The listing builds one solid part. Answer for the finished solid, in the listing's coordinates (mm). Coordinates: 2 decimals unless noted, no trailing zeros. Write each question's results on one line, items separated by ' | '. Start each with the question number.
(1) Straight lines are drawn through the part: L1, parallel to X at y = -35.5, z = 10; L2, parallel to Z at x = 11, y = -65; L3, parallel to X at y = -123.5, z = -11. For each, find the intervals that lie inside material, in ascending order.
(2) Given pin 1 (4 mm diameter, centred on x = 13.5, y = -122.5, fed in from -Z); pin 2 (6 mm diameter, centred on x = -12.5, y = -72.5, fed in from -Z); pin 3 (4 mm diameter, centred on x = -7.5, z = 0, fed in from +Y); pin 4 (10 mm diameter, centred on x = -12, y = -93.5, fed in from -Z), each flat-ended and moving along its own axis, determine where each tip first touches the part or whether it passes through.
(3) Determine the mould class of faces 1 (the face through (0, -69, 20)), 2 (the face through (-20, -85, 5)), 3 (the face through (0, -138, 19.5)) for opening direction X: +X half, -X half, draft (parallel to the pull), parting line (faces both ways), or undercut.
(4) The part is cut by section A-A, the plane z = -2.5. Count the separate pieces of the cut face and the enclosed holes in it, then the cut area to 3 significant figures.
```python
from build123d import *

# Parameters (mm, degrees)
F0_W      = 34
F0_H      = 1.332180649
F0_W_2    = 3
F0_H_2    = 30
F1_DEPTH  = 140
F3_DEPTH  = 50
F4_DEPTH  = 40
F5_T      = -0.5
F7_REACH  = 112.8020988928
F9_DEPTH  = 40
F11_DEPTH = 1000
F12_R     = 6.3171610822
F13_DEPTH = 140


# Not quite as in the source:
# - a feature names something its author has since deleted; it is built from what else it names


with BuildPart() as f1:
    # F0 (on Front) → F1 (new body)
    with BuildSketch(Plane.XZ):
        Polygon((20, 20), (17, 20), (17, 18.832180649), (17, 17.5), (17, 15), (20, 15), align=None)
        Polygon((15, 20), (-15, 20), (-17, 20), (-17, 18.832180649), (17, 18.832180649), (17, 20), align=None)
        with Locations((0, 18.1660903245)):
            Rectangle(F0_W, F0_H)
        Polygon((17, 17.5), (-17, 17.5), (-17, 15), (-17, -15), (-15, -15), (15, -15), (17, -15), (17, 15), align=None)
        Polygon((-18.5, 15), (-20, 15), (-20, -11.8550653383), (-20, -15), (-18.5, -15), (-18.5, -5.2632528394), (-18.5, -3.2632528394), (-18.5, 2.7367471606), (-18.5, 4.7367471606), align=None)
        with Locations((18.5, 0)):
            Rectangle(F0_W_2, F0_H_2)
        with BuildLine():
            Line((-15, -20), (15, -20))
            Line((15, -20), (15, -17.5))
            Line((15, -17.5), (11.391207267, -17.5))
            ThreePointArc((11.391207267, -17.5), (10.2485464886, -18.6426607784), (9.1058857102, -17.5))
            Line((9.1058857102, -17.5), (7.9234171988, -17.5))
            ThreePointArc((7.9234171988, -17.5), (5.948765669, -19.4746515298), (3.9741141393, -17.5))
            Line((3.9741141393, -17.5), (2.0740236579, -17.5))
            ThreePointArc((2.0740236579, -17.5), (0, -19.5740236579), (-2.0740236579, -17.5))
            Line((-2.0740236579, -17.5), (-3.9741141393, -17.5))
            ThreePointArc((-3.9741141393, -17.5), (-5.948765669, -19.4746515298), (-7.9234171988, -17.5))
            Line((-7.9234171988, -17.5), (-9.1058857102, -17.5))
            ThreePointArc((-9.1058857102, -17.5), (-10.2485464886, -18.6426607784), (-11.391207267, -17.5))
            Line((-11.391207267, -17.5), (-15, -17.5))
            Line((-15, -17.5), (-15, -20))
        make_face()
        Polygon((20, -20), (20, -15), (17, -15), (15, -15), (15, -17.5), (15, -20), align=None)
        Polygon((-17, -15), (-17, 15), (-18.5, 15), (-18.5, 4.7367471606), (-18.5, 2.7367471606), (-18.5, -3.2632528394), (-18.5, -5.2632528394), (-18.5, -15), align=None)
        Polygon((-15, -17.5), (-15, -15), (-16.767766953, -16.767766953), (-17.5, -17.5), (-15, -20), align=None)
        Polygon((-15, -15), (-17, -15), (-18.5, -15), (-20, -15), (-17.5, -17.5), (-16.767766953, -16.767766953), align=None)
        Polygon((-17, 18.832180649), (-17, 20), (-20, 20), (-20, 15), (-18.5, 15), (-17, 15), (-17, 17.5), align=None)
        Polygon((-17.5, -17.5), (-20, -15), (-20, -20), (-15, -20), align=None)
        with BuildLine():
            Line((3.9741141393, -17.5), (7.9234171988, -17.5))
            ThreePointArc((7.9234171988, -17.5), (5.948765669, -15.5253484702), (3.9741141393, -17.5))
        make_face()
        with BuildLine():
            ThreePointArc((3.9741141393, -17.5), (5.948765669, -19.4746515298), (7.9234171988, -17.5))
            Line((7.9234171988, -17.5), (3.9741141393, -17.5))
        make_face()
        with BuildLine():
            ThreePointArc((9.1058857102, -17.5), (10.2485464886, -18.6426607784), (11.391207267, -17.5))
            Line((11.391207267, -17.5), (9.1058857102, -17.5))
        make_face()
        with BuildLine():
            Line((9.1058857102, -17.5), (11.391207267, -17.5))
            ThreePointArc((11.391207267, -17.5), (10.2485464886, -16.3573392216), (9.1058857102, -17.5))
        make_face()
        with BuildLine():
            ThreePointArc((2.0740236579, -17.5), (0, -15.4259763421), (-2.0740236579, -17.5))
            Line((-2.0740236579, -17.5), (2.0740236579, -17.5))
        make_face()
        with BuildLine():
            Line((2.0740236579, -17.5), (-2.0740236579, -17.5))
            ThreePointArc((-2.0740236579, -17.5), (0, -19.5740236579), (2.0740236579, -17.5))
        make_face()
        with BuildLine():
            Line((-3.9741141393, -17.5), (-7.9234171988, -17.5))
            ThreePointArc((-7.9234171988, -17.5), (-5.948765669, -19.4746515298), (-3.9741141393, -17.5))
        make_face()
    extrude(amount=F1_DEPTH)


with BuildPart() as f1b:
    # F0 (on Front) → F1, piece 2 (new body)
    with BuildSketch(Plane.XZ):
        with BuildLine():
            ThreePointArc((-9.1058857102, -17.5), (-10.2485464886, -16.3573392216), (-11.391207267, -17.5))
            Line((-11.391207267, -17.5), (-9.1058857102, -17.5))
        make_face()
    extrude(amount=F1_DEPTH)


with BuildPart() as f3_tool:
    # F2 (on face) → F3 (new body)
    with BuildSketch(Plane.YZ.offset(20)):
        Polygon((0, 0), (-132.0431083441, -20), (0, -20), align=None)
    extrude(amount=-F3_DEPTH)


with BuildPart() as f1_1:
    add(f1.part)

    # F3: cut by f3_tool
    add(f3_tool.part, mode=Mode.SUBTRACT)



with BuildPart() as f1b_1:
    add(f1b.part)

    # F3: cut by f3_tool
    add(f3_tool.part, mode=Mode.SUBTRACT)


with BuildPart() as f1_2:
    add(f1_1.part)

    add(f1b_1.part)  # F4 merges F1b
    # F2 (on face) → F4 (join)
    with BuildSketch(Plane.YZ.offset(20)):
        Polygon((-133.1249161121, -12.857736984), (-132.0431083441, -20), (0, 0), (0, 7.3061197718), align=None)
        Polygon((-140, -20), (-132.0431083441, -20), (-133.1249161121, -12.857736984), (-140, -13.8990762821), align=None)
    extrude(amount=-F4_DEPTH)

    # F5
    f5_openings = [f1_2.faces().sort_by_distance(p)[0] for p in [
        (0, -140, 0),
    ]]
    offset(amount=F5_T, openings=f5_openings)

    f7_end = Plane(origin=(0, -66.021554172, -10), x_dir=(0, -0.988722747, -0.1497575692), z_dir=(0, 0.1497575692, -0.988722747))
    # F6 (on face) → F7 (join, up to a plane its end follows)
    with BuildSketch(Plane.XY.offset(20)):
        Polygon((0, -70), (-0.1507168075, -70), (0, -70.5315142328), (0.1507168075, -70), align=None)
        Polygon((0, -69.4684857672), (-0.1507168075, -70), (0, -70), (0.1507168075, -70), align=None)
        Polygon((0.1507168075, -70), (0, -70.5315142328), (19.6985663849, -140), (20, -140), align=None)
        Polygon((0, -70.5315142328), (-0.1507168075, -70), (-20, -140), (-19.6985663849, -140), align=None)
        Polygon((19.6985663849, 0), (0, -69.4684857672), (0.1507168075, -70), (20, 0), align=None)
        Polygon((-19.6985663849, 0), (-20, 0), (-0.1507168075, -70), (0, -69.4684857672), align=None)
    f7_long = extrude(amount=-F7_REACH, mode=Mode.PRIVATE)
    add(split(f7_long, bisect_by=f7_end, keep=Keep.BOTTOM, mode=Mode.PRIVATE))

    # F8 (on face) → F9 (join, through all)
    with BuildSketch(Plane.YZ.offset(20)):
        Polygon((-47.3704106226, 6.7672015175), (-46.6666666667, 6.6666666667), (-45.9831301115, 6.8619628253), (-46.6868740675, 6.9624976761), align=None)
        Polygon((-46.6868740675, 6.9624976761), (-45.9831301115, 6.8619628253), (0, 20), (-1.0556159339, 20), align=None)
        Polygon((-140, 20), (-47.3704106226, 6.7672015175), (-46.6868740675, 6.9624976761), (-137.9493903346, 20), align=None)
        Polygon((-45.9831301115, 6.8619628253), (-46.6666666667, 6.6666666667), (0, 0), (0, 0.2929442379), align=None)
        Polygon((-140, -19.6983954474), (-140, -20), (-46.6666666667, 6.6666666667), (-47.3704106226, 6.7672015175), align=None)
    extrude(amount=-F9_DEPTH)

    # F10 (on face) → F11 (cut)
    with BuildSketch(Plane(origin=(-20, 0, 0), x_dir=(0, -1, 0), z_dir=(-1, 0, 0))):
        Polygon((140, -20), (132.0431083441, -20), (132.0431083441, -21.8775942922), (142.034560442, -23.4243907034), (141.5658295155, -20), align=None)
    extrude(amount=-F11_DEPTH, mode=Mode.SUBTRACT)

    # F12 (on face) → F13 (cut, through all)
    with BuildSketch(Plane(origin=(0, 0, 0), x_dir=(-1, 0, 0), z_dir=(0, 1, 0))):
        with Locations((0, 10)):
            Circle(F12_R)
    extrude(amount=-F13_DEPTH, mode=Mode.SUBTRACT)


solid = f1_2.part
```
Established:
1) L1: x = -20 to -6.32, 6.32 to 20 | L2: z = -9.85 to -9.34, 1.43 to 1.73, 9.29 to 9.58, 19.5 to 20 | L3: x = -20 to -19.5, -15.32 to -15.02, 15.02 to 15.32, 19.5 to 20
2) pin 1: stops at z = -18.86 | pin 2: stops at z = -11.44 | pin 3: stops at y = 0 | pin 4: stops at z = -14.92
3) face 1: draft | face 2: -X half | face 3: undercut
4) separate pieces: 1 | enclosed holes: 6 | area: 366 mm^2
